Here's the drawing with two shaded views (mm, measured from the low corner). I have some questions. A direction names the side the tool comes from. Round coordinates to 2 decimals unless told otherwise and drop trailing zeros. Loops run counter-clockwise (first coordinate to the right, second up) from the corner with the lowest first, then second, coordinate; pieces in that order, holes last. Notation, with made-up numbers: (-24.5, 46) -> (-15.5, 46) arc R21 ccw to (-15.5, 83) -> close; hole circle Ø5 at (64, -16.75). An arc over 180 degrees is marked (long way). Write each question's results on one line, items separated by ' | '.
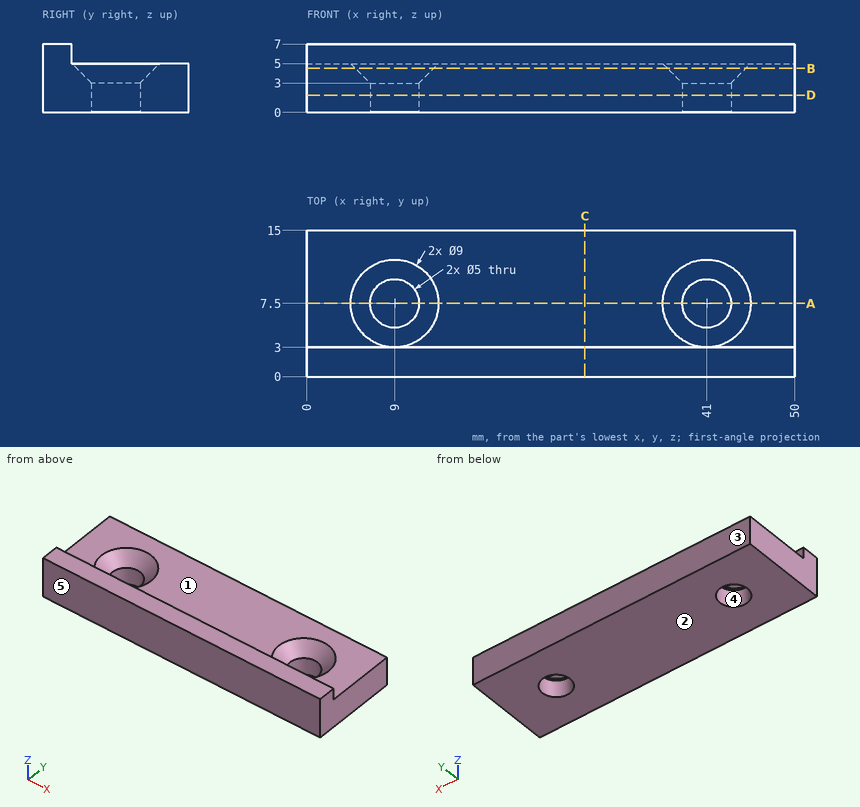
1. Will these pins go through, and if not, where does the flat tip stop? pin 1 (6 mm diameter, centred on x = 11.5, y = 7, fed in from +Z); pin 2 (4.5 mm diameter, centred on x = 41, y = 7.5, fed in from -Z); pin 3 (1.6 mm diameter, centred on x = 37.5, z = 6, fed in from +Y).
Final values:
pin 1: z = 5 | pin 2: through | pin 3: y = 3
2. On a 3-axis mill with a long thin cutter (end or side, diameter ignored), from which of +Z, -Z, +X, -X, +Y, -Y can I reach the whole of each face in a straight line? I mean the marked faces 1 and 2. Say none if no direction works.
Final values:
face 1: +Z, +X, -X, +Y | face 2: -Z, +X, -X, +Y, -Y
3. We'd pull the mould along Y, two halves only. Please class the marked faces 3, 4 and 5: pulls with the +Y half, pulls with the -Y half, needs draft (parallel to the pull), parting line crosses it, or undercut.
Final values:
face 3: pulls with the +Y half | face 4: undercut | face 5: pulls with the -Y half
4. If we section it at C-C (x = 28.5): List the corners of the cut face in (y, z) for me, then the cut area to 3 significant figures.
Final values:
outline: (0, 0) -> (15, 0) -> (15, 5) -> (3, 5) -> (3, 7) -> (0, 7) -> close | area: 81.0 mm2
5. If we section it at A-A (y = 7.5): List the corners of the cut face in (x, z) for me, then the cut area to 3 significant figures.
Final values:
outline: (0, 0) -> (6.5, 0) -> (6.5, 3) -> (4.5, 5) -> (0, 5) -> close; (11.5, 0) -> (38.5, 0) -> (38.5, 3) -> (36.5, 5) -> (13.5, 5) -> (11.5, 3) -> close; (43.5, 0) -> (50, 0) -> (50, 5) -> (45.5, 5) -> (43.5, 3) -> close | area: 192 mm2
6. If we section it at B-B (z = 4.5): List the corners of the cut face in (x, y) for me.
Final values:
outline: (0, 0) -> (50, 0) -> (50, 15) -> (0, 15) -> close; hole circle Ø8 at (9, 7.5); hole circle Ø8 at (41, 7.5)
7. If we section it at D-D (z = 1.75): List the corners of the cut face in (x, y) for me, then the cut area to 3 significant figures.
Final values:
outline: (0, 0) -> (50, 0) -> (50, 15) -> (0, 15) -> close; hole circle Ø5 at (9, 7.5); hole circle Ø5 at (41, 7.5) | area: 711 mm2
8. Please list where these lines run through material, in increasing order: line 1 (Z direction, x = 47, y = 3.75); line 2 (Y direction, x = 41, z = 1.65); line 3 (Y direction, x = 33.5, z = 5.5). Write a range as from..to.
Final values:
line 1: 0..5 | line 2: 0..5, 10..15 | line 3: 0..3
